from build123d import *

# Parameters (mm, degrees)
F0_W     = 133.841977
F0_H     = 113.085672
F1_DEPTH = 25.4
F2_R     = 8.131244
F3_DEPTH = 25.4
F5_D     = 6.35


with BuildPart() as f1:
    # F0 (on Front) → F1 (new body)
    with BuildSketch(Plane.XZ):
        with Locations((66.920988, 56.542836)):
            Rectangle(F0_W, F0_H)
    extrude(amount=F1_DEPTH)

    # F2 (on face) → F3 (cut)
    with BuildSketch(Plane.XZ.offset(25.4)):
        with Locations((24.086226, 81.72901)):
            Circle(F2_R)
    extrude(amount=-F3_DEPTH, mode=Mode.SUBTRACT)

    # F5 (through all)
    with Locations(Plane.XY.offset(113.085672)):
        with Locations((65.402642, -15.465394)):
            Hole(F5_D / 2)


solid = f1.part
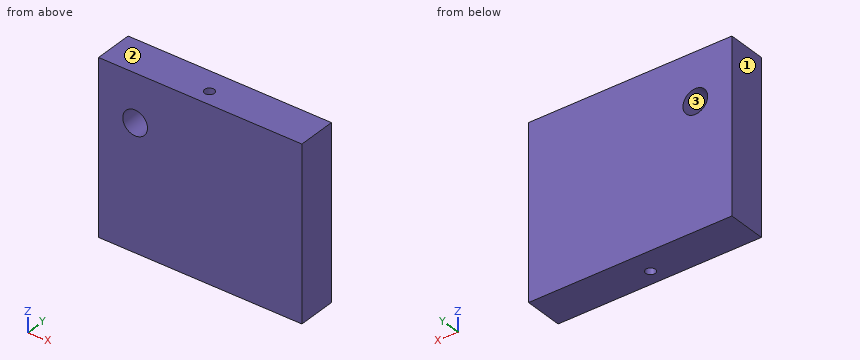
Verification items for the finished model (mm, model axes). Face numbers are marked on the shaded views. Give positions to 0.01 mm unless a question says otherwise; leave off trailing zeros. Order: outer loops, then holes, each group sorted by start corner. A loop starts at its lowest first (then second) coordinate and runs counter-clockwise, first axis right, second up. Notation, with made-up numbers: M 88.5,11 L 143.5,11 A17 cw 143.5,41 Z; hole C 61.5,51.25 d8. An arc over 180 degrees is marked long. Answer as a JSON object with one key per item and string values. Group by question number.
1) Depth check by flat-ended pin: pin 1 Ø12 at (x, y) = (32.5, -21) entering from -Z. Enter the tip coordinate at first touch or a pass-through.
2) Scan lines: line 1 along X through (y, z) = (-17.75, 79); line 2 along X through (y, z) = (-16, 73.5); line 3 along X through (y, z) = (-1.5, 88.5). Record each from-to range of solid material in increasing order. Write a range as [from, to].
3) Mould release check, pull along Z, two halves, no side actions. Record for the marked faces 1, 2 and 3: released by +Z, released by -Z, zero draft, split by the parting line, or undercut.
4) Cross-section at A-A (x = 64). Enter the section's corners in (y, z), then the cut area to 3 significant figures.
Result sheet:
{
 "1": {"pin 1": "stops at z = 0"},
 "2": {"line 1": "x = [0, 16.43], [31.75, 63.2], [67.61, 133.84]", "line 2": "x = [0, 62.27], [68.53, 133.84]", "line 3": "x = [0, 19.58], [28.59, 133.84]"},
 "3": {"face 1": "zero draft", "face 2": "released by +Z", "face 3": "undercut"},
 "4": {"outline": "M -25.4,0 L -18.31,0 L -18.31,113.09 L -25.4,113.09 Z; M -12.62,0 L 0,0 L 0,113.09 L -12.62,113.09 Z", "area": "2,230 mm2"}
}
